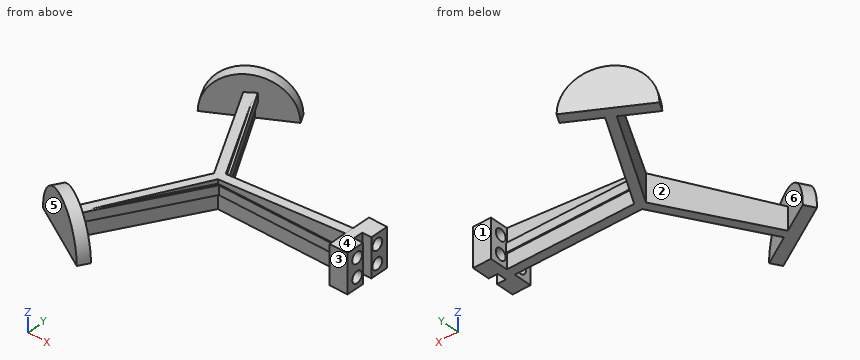
from build123d import *

# Parameters (mm, degrees)
F0_W      = 20
F0_H      = 17
F1_DEPTH  = 8
F2_W      = 4
F2_H      = 4.2
F3_DEPTH  = 17.001
F4_R      = 2.5
F5_DEPTH  = 8.001
F6_W      = 4
F6_H      = 6.5
F6_W_2    = 0.5
F6_H_2    = 4
F7_DEPTH  = 60
F9_DEPTH  = 17.001
F10_DEPTH = 50
F11_DEPTH = 50
F13_DEPTH = 47.8022701892
F14_DEPTH = 43.8022701892
F15_R     = 17.5
F16_DEPTH = 5
F17_R     = 17.5
F18_DEPTH = 5
F20_DEPTH = 108.9243937587


# Not quite as in the source:
# - a feature names something its author has since deleted; it is built from what else it names


with BuildPart() as f1:
    # F0 (on Right) → F1 (new body)
    with BuildSketch(Plane.YZ):
        Rectangle(F0_W, F0_H)
    extrude(amount=F1_DEPTH)

    # F2 (on face) → F3 (cut, through all)
    with BuildSketch(Plane.XY.offset(8.5)):
        with Locations((6, 0)):
            Rectangle(F2_W, F2_H)
    extrude(amount=-F3_DEPTH, mode=Mode.SUBTRACT)

    # F4 (on face) → F5 (cut, through all)
    with BuildSketch(Plane.YZ.offset(8)):
        with Locations((-5.1, 4)):
            Circle(F4_R)
        with Locations((5.1, 4)):
            Circle(F4_R)
        with Locations((-5.1, -4)):
            Circle(F4_R)
        with Locations((5.1, -4)):
            Circle(F4_R)
    extrude(amount=-F5_DEPTH, mode=Mode.SUBTRACT)

    # F6 (on Right) → F7 (join)
    with BuildSketch(Plane.YZ):
        with Locations((0, 5.25)):
            Rectangle(F6_W, F6_H)
        with Locations((2.25, 0)):
            Rectangle(F6_W_2, F6_H_2)
        Rectangle(F6_W, F6_H_2)
        with Locations((-2.25, 0)):
            Rectangle(F6_W_2, F6_H_2)
        with Locations((0, -5.25)):
            Rectangle(F6_W, F6_H)
    extrude(amount=-F7_DEPTH)

    # F8 (on face) → F9 (cut, through all)
    with BuildSketch(Plane.XY.offset(8.5)):
        Polygon((-60, -2.5), (-55.6698729811, -2.5), (-60, 0), align=None)
        Polygon((-60, 2.5), (-60, 0), (-55.6698729811, 2.5), align=None)
    extrude(amount=-F9_DEPTH, mode=Mode.SUBTRACT)

    # F10 (add): a face of the model
    f10_faces = [f1.faces().sort_by_distance(p)[0] for p in [
        (-58.1476678863, -1.0694444444, 0),
    ]]
    extrude(f10_faces, amount=F10_DEPTH)

    # F11 (add): a face of the model
    f11_faces = [f1.faces().sort_by_distance(p)[0] for p in [
        (-58.1476678863, 1.0694444444, 0),
    ]]
    extrude(f11_faces, amount=F11_DEPTH)

    # F12 (on face) → F13 (cut, through all)
    with BuildSketch(Plane.XZ.offset(2)):
        Polygon((0, 8.5), (-90.0749489665, 12.646025978), (-90.0749489665, 1.0502453661), align=None)
    extrude(amount=-F13_DEPTH, mode=Mode.SUBTRACT)

    # F12 (on face) → F14 (cut, through all)
    with BuildSketch(Plane.XZ.offset(2)):
        Polygon((0, 8.5), (-90.0749489665, 12.646025978), (-90.0749489665, 1.0502453661), align=None)
    extrude(amount=F14_DEPTH, mode=Mode.SUBTRACT)

    # F15 (on face) → F16 (join)
    with BuildSketch(Plane(origin=(-40, -69.2820323028, 0), x_dir=(0.8660254038, -0.5, 0), z_dir=(-0.5, -0.8660254038, 0))):
        with Locations((-49.9615242271, -8.5)):
            Circle(F15_R)
    extrude(amount=F16_DEPTH)

    # F17 (on face) → F18 (join)
    with BuildSketch(Plane(origin=(-40, 69.2820323028, 0), x_dir=(-0.8660254038, -0.5, 0), z_dir=(-0.5, 0.8660254038, 0))):
        with Locations((49.9615242271, -8.5)):
            Circle(F17_R)
    extrude(amount=F18_DEPTH)

    # F19 (on face) → F20 (cut, through all)
    with BuildSketch(Plane.YZ.offset(8)):
        Polygon((63.882611692, -8.5), (0, -8.5), (-60.1151846349, -8.5), (-60.0160695612, -29.4797774404), (63.882611692, -28.5877082497), align=None)
    extrude(amount=-F20_DEPTH, mode=Mode.SUBTRACT)


solid = f1.part
Verification items for the finished model (mm, model axes). Face numbers are marked on the shaded views. A direction names the side the tool comes from. Coordinates: 2 decimals unless noted, no trailing zeros. Order: outer loops, then holes, each group sorted by start corner. A loop starts at its lowest first (then second) coordinate and runs counter-clockwise, first axis right, second up. Notation, with made-up numbers: (37.25, 22.25) -> (62.25, 22.25) arc R32 ccw to (62.25, 52.25) -> close; hole circle Ø10 at (9.25, -19). An arc over 180 degrees is marked (long way). Put each result on its own line as item: value. Start each with the question number.
1. Cross-section at B-B, the plane x = -30. Record the boundary of the cut face in (y, z).
2. Go/stop test with flat-tipped pins: pin 1 Ø6.5 at (y, z) = (-5.1, -4) entering from -X; pin 2 Ø6 at (y, z) = (5.1, -4) entering from +X; pin 3 Ø2 at (x, z) = (-25.5, -5.5) entering from +Y; pin 4 Ø4 at (x, z) = (2, 1) entering from +Y. Record where each tip stops, or that it passes through.
3. Access from +Z, -Z, +X, -X, +Y, -Y to the whole of each face (thin tool, end or side, straight path). Record for the marked faces 1, 2 and 3.
4. Mould release check, pull along X, two halves, no side actions. Record for the marked faces 4, 5 and 6: released by +X, released by -X, zero draft, split by the parting line, or undercut.
5. Material ranges on L1, parallel to Z at x = 6.5, y = 5.1; L2, parallel to Y at x = 2.5, z = 5; L3, parallel to Y at x = -79, z = -1.5, recorded low to high. Write a range as [from, to].
6. Cross-section at A-A, the plane y = -5.1. Record the boundary of the cut face in (x, z).
7. Cross-section at C-C, the plane x = -46. Record the boundary of the cut face in (y, z), then the cut area to 3 significant figures.
Computed:
1. outline: (-2.5, -2) -> (-2, -2) -> (-2, -8.5) -> (2, -8.5) -> (2, -2) -> (2.5, -2) -> (2.5, 2) -> (2, 2) -> (2, 6.02) -> (-2, 6.02) -> (-2, 2) -> (-2.5, 2) -> close
2. pin 1: x = -64.82
2. pin 2: x = 8
2. pin 3: y = 2
2. pin 4: y = 10
3. face 1: +Z, -Z, +X, +Y
3. face 2: +Z, -Z
3. face 3: +Z, -Z, +X, -Y
4. face 4: zero draft
4. face 5: released by -X
4. face 6: undercut
5. L1: [-8.5, -6.5], [-1.5, 1.5], [6.5, 8.5]
5. L2: [-10, -7.39], [-2.81, 2.81], [7.39, 10]
5. L3: [-52.54, -46.77], [-42.91, -32.91], [32.91, 42.91], [46.77, 52.54]
6. outline: (-62.94, -8.5) -> (-58.33, -8.5) -> (-58.33, -2) -> (-57.17, -2) -> (-57.17, 2) -> (-58.33, 2) -> (-58.33, 3.68) -> (-62.94, 3.29) -> close; (0, -8.5) -> (8, -8.5) -> (8, -6.5) -> (0, -6.5) -> close; (0, -1.5) -> (8, -1.5) -> (8, 1.5) -> (0, 1.5) -> close; (0, 6.5) -> (8, 6.5) -> (8, 8.5) -> (0, 8.5) -> close
7. outline: (-2.5, -2) -> (-2, -2) -> (-2, -8.5) -> (2, -8.5) -> (2, -2) -> (2.5, -2) -> (2.5, 2) -> (2, 2) -> (2, 4.7) -> (-2, 4.7) -> (-2, 2) -> (-2.5, 2) -> close
7. area: 56.8 mm2
